Autodesk Inventor part; units mm, degrees
ref_plane "YZ Plane" through (0, 0, 0) normal (1, 0, 0) x (0, 1, 0)
ref_plane "XZ Plane" through (0, 0, 0) normal (0, 1, 0) x (-1, 0, 0)
ref_plane "XY Plane" through (0, 0, 0) normal (0, 0, 1) x (1, 0, 0)
sketch "スケッチ1" plane through (0, 0, 0) normal (0, 0, 1) x (1, 0, 0)
  line L0 (0, 0) -> (1.5, 0)
  line L1 (1.5, 0) -> (1.5, 6)
  line L2 (1.5, 6) -> (2.6, 6)
  line L3 (2.6, 6) -> (2.6, 7.2) construction
  line L4 (2.6, 7.2) -> (0, 7.2)
  line L5 (0, 7.2) -> (0, 0)
  line L6 (0, -5.542) -> (0, 0) construction
  arc A0 (2.6, 6) -> (2.6, 7.2) centre (1.8, 6.6) ccw
  line L7 (2.8, 9.0711) -> (2.8, 6.853) construction
  dimension "d0" = 3
  dimension "d1" = 6
  dimension "d2" = 5.2
  dimension "d3" = 1.2
  dimension "d13" = 5.6
revolve "回転1" add sketch "スケッチ1" angle 360 about axis through (0, -5.542, 0) along (0, 1, 0)
sketch "スケッチ2" plane through (0, 7.2, 0) normal (0, 1, 0) x (1, 0, 0)
  line L0 (1.1547, 0) -> (0.5774, -1)
  line L1 (0.5774, -1) -> (-0.5774, -1)
  line L2 (-0.5774, -1) -> (-1.1547, 0)
  line L3 (-1.1547, 0) -> (-0.5774, 1)
  line L4 (-0.5774, 1) -> (0.5774, 1)
  line L5 (0.5774, 1) -> (1.1547, 0)
  line L6 (1.1547, 0) -> (-1.1547, 0) construction
  point P0 (0, 0)
  point P1 (0, 0)
  dimension "d5" = 2
extrude "押し出し1" cut sketch "スケッチ2" against normal blind 1
fillet "フィレット1" radius 0.4 1 edges at (-2.6, 7.2, 0)
fillet "フィレット1" radius 0.3 1 edges at (-2.6, 6, 0)
chamfer "面取り1" distance 0.25 angle 45 1 edges at (-1.5, 0, 0)
properties part number "10_051_LOW_HEAD_CAP_BOLT_M3X6_R1"
Could you check a few things on this model? Use its own coordinates, in mm. A direction names the side the tool comes from. Give positions to 0.01 mm unless a question says otherwise; leave off trailing zeros. Loops run counter-clockwise (first coordinate to the right, second up) from the corner with the lowest first, then second, coordinate; pieces in that order, holes last. Notation, with made-up numbers: (25.25, 53) - (61.25, 53) arc R6 cw to (61.25, 58) - close; hole circle Ø4 at (-7.75, -15). An arc over 180 degrees is marked (long way). Answer in a Markdown table with one row per item. Add a question column.
Q1. Which directions (+Z, -Z, +X, -X, +Y, -Y) give clear straight access to the entire face, cutting with the end or side of a thin tool? Please do faces 4 (the face through (-0.87, 6.71, -0.49)), 5 (the face through (0, 0, 0)).
Q2. Please list where these lines run through material, in increasing order: L1, parallel to Y at x = 0.85, z = 1.4; L2, parallel to X at y = 0.5, z = 0.05; L3, parallel to Y at x = -0.8, z = -0.5. Write a range as from..to.
Q3. If we section it at A-A (y = 5.75): List the corners of the cut face in (x, z) for me, plus the area to 3 significant figures.
Q4. For pin 1 (1.5 mm diameter, centred on x = -1, y = 6.5, fed in from -Z); pin 2 (3 mm diameter, centred on y = 3, z = 0.5, fed in from -X), each with a flat end and sliding along its axis, tell me the tip position at first contact or that it passes through.
Q5. We'd pull the mould along X, two halves only. Please class faces 1 (the face through (0.87, 6.71, 0.49)), 2 (the face through (1, 7.2, 1)), 3 (the face through (-1.5, 3.17, -0.07)): +X half, -X half, draft (parallel to the pull), parting line (faces both ways), or undercut.
The answers:
| question | item | result |
|---|---|---|
| 1 | face 4 | +Y |
| 1 | face 5 | +Z, -Z, +X, -X, -Y |
| 2 | L1 | y = 6..7.2 |
| 2 | L2 | x = -1.5..1.5 |
| 2 | L3 | y = 0..6.2 |
| 3 | outline | circle Ø3 at (0, 0) |
| 3 | area | 7.07 mm^2 |
| 4 | pin 1 | stops at z = -2.79 |
| 4 | pin 2 | stops at x = -1.5 |
| 5 | face 1 | undercut |
| 5 | face 2 | draft |
| 5 | face 3 | parting line |
